```python
from build123d import *

# Parameters (mm, degrees)
BOSS_EXTRUDE1_DEPTH = 64
FILLET1_R           = 1
CUT_EXTRUDE1_DEPTH  = 65
FILLET2_R           = 0.5
FILLET3_R           = 0.25


with BuildPart() as part:
    # Sketch3 → Boss-Extrude1 (new body)
    with BuildSketch(Plane(origin=(0, 0, 0), x_dir=(1, 0, 0), z_dir=(0, 1, 0))):
        with BuildLine():
            Line((7, 18.5), (7, 19.5))
            ThreePointArc((7, 19.5), (6.646446609, 19.646446609), (6.5, 20))
            Line((6.5, 20), (0, 20))
            Line((0, 20), (0, 13.5))
            ThreePointArc((0, 13.5), (0.353553391, 13.353553391), (0.5, 13))
            Line((0.5, 13), (1.5, 13))
            Line((1.5, 13), (1.5, 16))
            Line((1.5, 16), (3, 16))
            Line((3, 16), (5.5, 13.5))
            Line((5.5, 13.5), (5.5, 10.5))
            Line((5.5, 10.5), (6, 10))
            Line((6, 10), (5.5, 9.5))
            Line((5.5, 9.5), (5.5, 6.5))
            Line((5.5, 6.5), (3, 4))
            Line((3, 4), (1.5, 4))
            Line((1.5, 4), (1.5, 7))
            Line((1.5, 7), (0.5, 7))
            ThreePointArc((0.5, 7), (0.353553391, 6.646446609), (0, 6.5))
            Line((0, 6.5), (0, 0))
            Line((0, 0), (6.5, 0))
            ThreePointArc((6.5, 0), (6.646446609, 0.353553391), (7, 0.5))
            Line((7, 0.5), (7, 1.5))
            Line((7, 1.5), (4, 1.5))
            Line((4, 1.5), (4, 3))
            Line((4, 3), (6.5, 5.5))
            Line((6.5, 5.5), (9.5, 5.5))
            Line((9.5, 5.5), (10, 6))
            Line((10, 6), (10.5, 5.5))
            Line((10.5, 5.5), (13.5, 5.5))
            Line((13.5, 5.5), (16, 3))
            Line((16, 3), (16, 1.5))
            Line((16, 1.5), (13, 1.5))
            Line((13, 1.5), (13, 0.5))
            ThreePointArc((13, 0.5), (13.353553391, 0.353553391), (13.5, 0))
            Line((13.5, 0), (20, 0))
            Line((20, 0), (20, 6.5))
            ThreePointArc((20, 6.5), (19.646446609, 6.646446609), (19.5, 7))
            Line((19.5, 7), (18.5, 7))
            Line((18.5, 7), (18.5, 4))
            Line((18.5, 4), (17, 4))
            Line((17, 4), (14.5, 6.5))
            Line((14.5, 6.5), (14.5, 9.5))
            Line((14.5, 9.5), (14, 10))
            Line((14, 10), (14.5, 10.5))
            Line((14.5, 10.5), (14.5, 13.5))
            Line((14.5, 13.5), (17, 16))
            Line((17, 16), (18.5, 16))
            Line((18.5, 16), (18.5, 13))
            Line((18.5, 13), (19.5, 13))
            ThreePointArc((19.5, 13), (19.646446609, 13.353553391), (20, 13.5))
            Line((20, 13.5), (20, 20))
            Line((20, 20), (13.5, 20))
            ThreePointArc((13.5, 20), (13.353553391, 19.646446609), (13, 19.5))
            Line((13, 19.5), (13, 18.5))
            Line((13, 18.5), (16, 18.5))
            Line((16, 18.5), (16, 17))
            Line((16, 17), (13.5, 14.5))
            Line((13.5, 14.5), (10.5, 14.5))
            Line((10.5, 14.5), (10, 14))
            Line((10, 14), (9.5, 14.5))
            Line((9.5, 14.5), (6.5, 14.5))
            Line((6.5, 14.5), (4, 17))
            Line((4, 17), (4, 18.5))
            Line((4, 18.5), (7, 18.5))
        make_face()
    extrude(amount=BOSS_EXTRUDE1_DEPTH)

    # Fillet1
    fillet1_edges = [part.edges().sort_by_distance(p)[0] for p in [
        (20, 32, 0),
        (0, 32, 0),
        (0, 32, -20),
        (20, 32, -20),
    ]]
    fillet(fillet1_edges, radius=FILLET1_R)

    # Sketch4 → Cut-Extrude1 (cut, through all)
    with BuildSketch(Plane(origin=(0, 64, 0), x_dir=(1, 0, 0), z_dir=(0, 1, 0))):
        with BuildLine():
            Line((10, 11), (11.195582496, 12.195582496))
            ThreePointArc((11.195582496, 12.195582496), (10, 12.5), (8.804417504, 12.195582496))
            Line((8.804417504, 12.195582496), (10, 11))
        make_face()
        with BuildLine():
            ThreePointArc((12.195582496, 11.195582496), (11.767766953, 11.767766953), (11.195582496, 12.195582496))
            Line((11.195582496, 12.195582496), (10, 11))
            Line((10, 11), (11, 10))
            Line((11, 10), (12.195582496, 11.195582496))
        make_face()
        with BuildLine():
            Line((9, 10), (10, 11))
            Line((10, 11), (8.804417504, 12.195582496))
            ThreePointArc((8.804417504, 12.195582496), (8.232233047, 11.767766953), (7.804417504, 11.195582496))
            Line((7.804417504, 11.195582496), (9, 10))
        make_face()
        Polygon((11, 10), (10, 11), (9, 10), (10, 9), align=None)
        with BuildLine():
            Line((7.804417504, 8.804417504), (9, 10))
            Line((9, 10), (7.804417504, 11.195582496))
            ThreePointArc((7.804417504, 11.195582496), (7.5, 10), (7.804417504, 8.804417504))
        make_face()
        with BuildLine():
            Line((10, 9), (9, 10))
            Line((9, 10), (7.804417504, 8.804417504))
            ThreePointArc((7.804417504, 8.804417504), (8.232233047, 8.232233047), (8.804417504, 7.804417504))
            Line((8.804417504, 7.804417504), (10, 9))
        make_face()
        with BuildLine():
            Line((11.195582496, 7.804417504), (10, 9))
            Line((10, 9), (8.804417504, 7.804417504))
            ThreePointArc((8.804417504, 7.804417504), (10, 7.5), (11.195582496, 7.804417504))
        make_face()
        with BuildLine():
            Line((12.195582496, 8.804417504), (11, 10))
            Line((11, 10), (10, 9))
            Line((10, 9), (11.195582496, 7.804417504))
            ThreePointArc((11.195582496, 7.804417504), (11.767766953, 8.232233047), (12.195582496, 8.804417504))
        make_face()
        with BuildLine():
            ThreePointArc((12.5, 10), (12.422700584, 10.616864556), (12.195582496, 11.195582496))
            Line((12.195582496, 11.195582496), (11, 10))
            Line((11, 10), (12.195582496, 8.804417504))
            ThreePointArc((12.195582496, 8.804417504), (12.422700584, 9.383135444), (12.5, 10))
        make_face()
        with BuildLine():
            ThreePointArc((8.804417504, 7.804417504), (8.232233047, 8.232233047), (7.804417504, 8.804417504))
            Line((7.804417504, 8.804417504), (7, 8))
            Line((7, 8), (8, 7))
            Line((8, 7), (8.804417504, 7.804417504))
        make_face()
        with BuildLine():
            Line((13, 8), (12.195582496, 8.804417504))
            ThreePointArc((12.195582496, 8.804417504), (11.767766953, 8.232233047), (11.195582496, 7.804417504))
            Line((11.195582496, 7.804417504), (12, 7))
            Line((12, 7), (13, 8))
        make_face()
        with BuildLine():
            Line((13, 12), (12, 13))
            Line((12, 13), (11.195582496, 12.195582496))
            ThreePointArc((11.195582496, 12.195582496), (11.767766953, 11.767766953), (12.195582496, 11.195582496))
            Line((12.195582496, 11.195582496), (13, 12))
        make_face()
        with BuildLine():
            ThreePointArc((7.804417504, 11.195582496), (8.232233047, 11.767766953), (8.804417504, 12.195582496))
            Line((8.804417504, 12.195582496), (8, 13))
            Line((8, 13), (7, 12))
            Line((7, 12), (7.804417504, 11.195582496))
        make_face()
    extrude(amount=-CUT_EXTRUDE1_DEPTH, mode=Mode.SUBTRACT)

    # Fillet2
    fillet2_edges = [part.edges().sort_by_distance(p)[0] for p in [
        (18.5, 32, -13),
        (18.5, 32, -16),
        (14.5, 32, -10.5),
        (14.5, 32, -9.5),
        (18.5, 32, -4),
        (18.5, 32, -7),
        (13, 32, -1.5),
        (16, 32, -1.5),
        (10.5, 32, -5.5),
        (9.5, 32, -5.5),
        (4, 32, -1.5),
        (7, 32, -1.5),
        (1.5, 32, -7),
        (1.5, 32, -4),
        (5.5, 32, -9.5),
        (5.5, 32, -10.5),
        (1.5, 32, -16),
        (1.5, 32, -13),
        (7, 32, -18.5),
        (4, 32, -18.5),
        (9.5, 32, -14.5),
        (10.5, 32, -14.5),
        (16, 32, -18.5),
        (13, 32, -18.5),
    ]]
    fillet(fillet2_edges, radius=FILLET2_R)

    # Fillet3
    fillet3_edges = [part.edges().sort_by_distance(p)[0] for p in [
        (7, 32, -12),
        (8, 32, -13),
        (12, 32, -13),
        (13, 32, -12),
        (13, 32, -8),
        (12, 32, -7),
        (8, 32, -7),
        (7, 32, -8),
    ]]
    fillet(fillet3_edges, radius=FILLET3_R)


solid = part.part
```
Geometry check sheet. Reference: the model listing, model coordinates, mm. A direction names the side the tool comes from. Round coordinates to 2 decimals unless told otherwise and drop trailing zeros. Put each result on its own line as item: value.
1) Access from +Z, -Z, +X, -X, +Y, -Y to the whole of each face (thin tool, end or side, straight path). Record for faces 4 (the face through (12, 32, -14.5)), 5 (the face through (0, 32, -16)).
Recorded:
face 4: +Y, -Y
face 5: +Z, -Z, -X, +Y, -Y
2) Depth check by flat-ended pin: P1, Ø1.4, axis at x = 8, y = 39.5, coming from the +Z side; P2, Ø2, axis at x = 9.5, z = -17.5, coming from the -Y side. Enter the tip coordinate at first touch or a pass-through.
Recorded:
P1: stops at z = -5.5
P2: passes through
3) Release check for a two-part mould opening along X. For faces 1 (the face through (4, 32, 0)), 2 (the face through (14, 32, -18.5)), 3 (the face through (0, 32, -4)) record: pulls with the +X half, pulls with the -X half, needs draft (parallel to the pull), parting line crosses it, or undercut.
Recorded:
face 1: needs draft
face 2: undercut
face 3: pulls with the -X half
4) Thickness scan on probe 1 along Z at (x, y) = (1, 39.5); probe 2 along X at (y, z) = (25.5, -5.25); probe 3 along Z at (x, y) = (15.25, 32.5). Record the ranges inside material, lowest first. Write a range as from..to.
Recorded:
probe 1: z = -20..-13, -7..0
probe 2: x = 0..1.5, 4.25..6.25, 13.75..15.75, 18.5..20
probe 3: z = -20..-18.5, -16.25..-14.25, -5.75..-3.75, -1.5..0
